For this review, take the finished solid that the model builds, in its own axes (mm). Face numbers are marked on the shaded views. A direction names the side the tool comes from. Coordinates: 2 decimals unless noted, no trailing zeros. Loops run counter-clockwise (first coordinate to the right, second up) from the corner with the lowest first, then second, coordinate; pieces in that order, holes last. Notation, with made-up numbers: M 17.25,33.5 L 23.25,33.5 A15 cw 23.25,42.5 Z; hole C 71,26.5 d2. An arc over 180 degrees is marked long. Put each result on its own line as item: value.
```python
from build123d import *

# Parameters (mm, degrees)
F0_W     = 50.8
F0_H     = 50.8
F1_DEPTH = 3.175
F2_R     = 3.175
F3_DEPTH = 50.8


with BuildPart() as f1:
    # F0 (on Top) → F1 (new body)
    with BuildSketch(Plane.XY):
        Rectangle(F0_W, F0_H)
    extrude(amount=F1_DEPTH)

    # F2 (on face) → F3 (join, through all)
    with BuildSketch(Plane(origin=(-25.4, 0, 0), x_dir=(0, -1, 0), z_dir=(-1, 0, 0))):
        with Locations((0, 1.5875)):
            Circle(F2_R)
    extrude(amount=-F3_DEPTH)


solid = f1.part
```
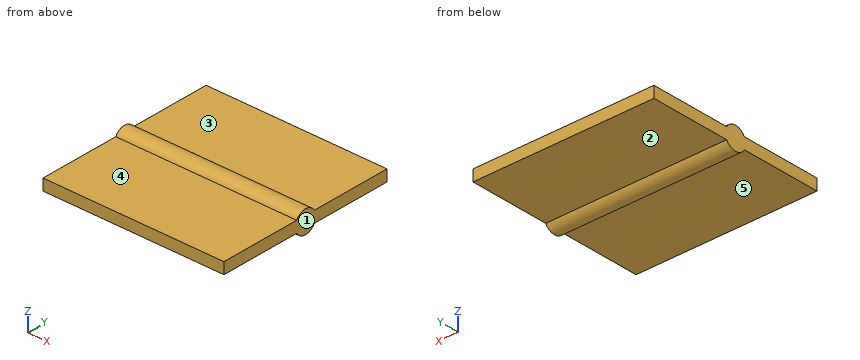
(1) Add section B-B (y = 15). Write out the cut boundary in (x, z) (3 decimals).
Determined:
outline: M -25.4,0 L 25.4,0 L 25.4,3.175 L -25.4,3.175 Z
(2) Wall thickness on line 1 along Z through (x, y) = (-16.5, 14) (3 decimals); line 2 along Y through (x, z) = (-5, -0.5); line 3 along Y through (x, z) = (20.5, 4): over which ranges is each line inside the solid? List them lowest first. Write a range as [from, to].
Determined:
line 1: z = [0, 3.175]
line 2: y = [-2.39, 2.39]
line 3: y = [-2.06, 2.06]
(3) Add section C-C (y = -1.5). Write out the cut boundary in (x, z).
Determined:
outline: M -25.4,-1.21 L 25.4,-1.21 L 25.4,4.39 L -25.4,4.39 Z
(4) For pin 1 (8 mm diameter, centred on x = -17, y = 7.5, fed in from +Z) (3 decimals); pin 2 (3 mm diameter, centred on x = -11, y = 15.5, fed in from -Z); pin 3 (25 mm diameter, centred on x = 3, y = -10.5, fed in from +Z); pin 4 (2 mm diameter, centred on x = -10.5, y = -2.5, fed in from -Z), all flat-tipped, find the tip position at first contact; note any pin that passes through.
Determined:
pin 1: stops at z = 3.175
pin 2: stops at z = 0
pin 3: stops at z = 4.76
pin 4: stops at z = -1.21
(5) Tool access review of the marked faces 1, 2, 3, 4 and 5: name each direction out of +Z, -Z, +X, -X, +Y, -Y from which nothing blocks a thin tool from reaching the whole face with its end or side.
Determined:
face 1: +Z, -Z, +X, +Y, -Y
face 2: -Z, +X, -X, +Y
face 3: +Z, +X, -X, +Y
face 4: +Z, +X, -X, -Y
face 5: -Z, +X, -X, -Y
